Build history of the part. All positions in model axes, mm. A direction names the side the tool comes from. Round coordinates to 2 decimals unless told otherwise and drop trailing zeros. Order: outer loops, then holes, each group sorted by start corner. A loop starts at its lowest first (then second) coordinate and runs counter-clockwise, first axis right, second up. Notation, with made-up numbers: (55.25, 58.5) -> (62.25, 58.5) arc R27 ccw to (62.25, 86.5) -> close; hole circle Ø2 at (63.25, 68). An arc over 180 degrees is marked (long way). Write item = value, one per line.
from build123d import *

# Parameters (mm, degrees)
F1_DEPTH  = 125
F2_R      = 26.25
F3_DEPTH  = 25
F4_W      = 97.6103432477
F4_H      = 17.1008444879
F5_DEPTH  = 22.5
F7_DEPTH  = 223
F9_DEPTH  = 25
F10_R     = 5
F12_DEPTH = 25


with BuildPart() as f1:
    # F0 (on Right) → F1 (new body, symmetric)
    with BuildSketch(Plane.YZ):
        with BuildLine():
            Line((150.9032388148, 0), (0, 0))
            Line((0, 0), (0, -3.0000018725))
            Line((0, -3.0000018725), (150.9032388148, -3.0000018725))
            ThreePointArc((150.9032388148, -3.0000018725), (177.0839005299, 9.9108717028), (182.778792891, 38.541028973))
            Line((182.778792891, 38.541028973), (157.1357605543, 134.2421285136))
            ThreePointArc((157.1357605543, 134.2421285136), (145.53968371, 148.6905408156), (127.0530008041, 149.9022220292))
            Line((127.0530008041, 149.9022220292), (-35.6771693401, 90.6732838797))
            ThreePointArc((-35.6771693401, 90.6732838797), (-44.8528287691, 91.0739018222), (-51.0577201094, 97.8453524901))
            Line((-51.0577201094, 97.8453524901), (-52.767820826, 102.543815594))
            Line((-52.767820826, 102.543815594), (-55.586900448, 101.5177545236))
            Line((-55.586900448, 101.5177545236), (-53.8767997313, 96.8192914196))
            ThreePointArc((-53.8767997313, 96.8192914196), (-46.1206843457, 88.354976764), (-34.6511082697, 87.8542042577))
            Line((-34.6511082697, 87.8542042577), (128.0790618745, 147.0831424073))
            ThreePointArc((128.0790618745, 147.0831424073), (144.1544370057, 146.0295066551), (154.2379812668, 133.4656708936))
            Line((154.2379812668, 133.4656708936), (179.8810136034, 37.7645713531))
            ThreePointArc((179.8810136034, 37.7645713531), (174.7038390235, 11.7371571297), (150.9032388148, 0))
        make_face()
    extrude(amount=F1_DEPTH, both=True)

    # F2 (on face) → F3 (cut)
    with BuildSketch(Plane(origin=(0, 180.1701926471, 48.2764576199), x_dir=(-1, 0, 0), z_dir=(0, 0.9659258263, 0.2588190451))):
        with Locations((0, 35)):
            Circle(F2_R)
    extrude(amount=-F3_DEPTH, mode=Mode.SUBTRACT)

    # F4 (on face) → F5 (cut, symmetric)
    with BuildSketch(Plane(origin=(0, -33.3152677142, 91.5329457678), x_dir=(1, 0, 0), z_dir=(0, -0.3420201433, 0.9396926208))):
        with Locations((93.8051716238, -11.063905455)):
            Rectangle(F4_W, F4_H)
        with Locations((-93.8051716238, -11.063905455)):
            Rectangle(F4_W, F4_H)
    extrude(amount=F5_DEPTH, both=True, mode=Mode.SUBTRACT)

    # F6 (on face) → F7 (cut)
    with BuildSketch(Plane(origin=(0, -33.3152677142, 91.5329457678), x_dir=(1, 0, 0), z_dir=(0, -0.3420201433, 0.9396926208))):
        with BuildLine():
            Line((-124.9454884285, 11.1526290369), (-110, 170.6603467676))
            Line((-110, 170.6603467676), (-107.1620267497, 200.9489946296))
            Line((-107.1620267497, 200.9489946296), (-152.5835648179, 200.9489946296))
            Line((-152.5835648179, 200.9489946296), (-152.5835648179, -22.4528324986))
            Line((-152.5835648179, -22.4528324986), (-112.5, -22.4528324986))
            Line((-112.5, -22.4528324986), (-112.5, -2.5134832111))
            ThreePointArc((-112.5, -2.5134832111), (-121.74192629, 1.5700568176), (-124.9454884285, 11.1526290369))
        make_face()
        with BuildLine():
            Line((112.5, -2.5134832111), (112.5, -22.4528324986))
            Line((112.5, -22.4528324986), (152.5835648179, -22.4528324986))
            Line((152.5835648179, -22.4528324986), (152.5835648179, 200.9489946296))
            Line((152.5835648179, 200.9489946296), (107.1620267497, 200.9489946296))
            Line((107.1620267497, 200.9489946296), (110, 170.6603467676))
            Line((110, 170.6603467676), (124.9454884285, 11.1526290369))
            ThreePointArc((124.9454884285, 11.1526290369), (121.74192629, 1.5700568176), (112.5, -2.5134832111))
        make_face()
    extrude(amount=-F7_DEPTH, mode=Mode.SUBTRACT)

    # F8 (on face) → F9 (cut)
    with BuildSketch(Plane(origin=(0, 0, -3.0000018725), x_dir=(1, 0, 0), z_dir=(0, 0, -1))):
        with BuildLine():
            ThreePointArc((-124.7078686175, -15), (-120.3144703352, -4.3933982822), (-109.7078686175, 0))
            Line((-109.7078686175, 0), (-109.7078686175, 1.8405353206))
            Line((-109.7078686175, 1.8405353206), (-139.135748148, 2.5484173093))
            Line((-139.135748148, 2.5484173093), (-139.135748148, -15))
            Line((-139.135748148, -15), (-124.7078686175, -15))
        make_face()
        with BuildLine():
            Line((109.7078686175, 1.8405353206), (109.7078686175, 0))
            ThreePointArc((109.7078686175, 0), (120.3144703352, -4.3933982822), (124.7078686175, -15))
            Line((124.7078686175, -15), (139.135748148, -15))
            Line((139.135748148, -15), (139.135748148, 2.5484173093))
            Line((139.135748148, 2.5484173093), (109.7078686175, 1.8405353206))
        make_face()
    extrude(amount=-F9_DEPTH, mode=Mode.SUBTRACT)

    # F10
    f10_edges = [f1.edges().sort_by_distance(p)[0] for p in [
        (-45, -35.164139, 89.263744),
        (45, -35.164139, 89.263744),
        (45, -54.177361, 102.030785),
        (-45, -54.177361, 102.030785),
    ]]
    fillet(f10_edges, radius=F10_R)

    # F11 (on face) → F12 (cut)
    with BuildSketch(Plane(origin=(0, -33.3152677142, 91.5329457678), x_dir=(1, 0, 0), z_dir=(0, -0.3420201433, 0.9396926208))):
        with BuildLine():
            ThreePointArc((-9.5571116428, 97.9430625287), (-8.0445828135, 89.0599084724), (0, 85))
            ThreePointArc((0, 85), (8.0445828135, 89.0599084724), (9.5571116428, 97.9430625287))
            add(Edge.make_bspline(
                [(0.2464486877, 118.196647138), (1.8167264508, 108.9800336214), (7.4531598076, 104.7753001668), (9.5571116428, 97.9430625287)],
                knots=[1.4245432684, 1.4245432684, 1.4245432684, 1.4245432684, 24.0384457394, 24.0384457394, 24.0384457394, 24.0384457394], degree=3))
            ThreePointArc((0.2464486877, 118.196647138), (0, 118.4046585168), (-0.2464486877, 118.196647138))
            add(Edge.make_bspline(
                [(-0.2464486877, 118.196647138), (-1.8167264508, 108.9800336214), (-7.4531598076, 104.7753001668), (-9.5571116428, 97.9430625287)],
                knots=[1.4245432684, 1.4245432684, 1.4245432684, 1.4245432684, 24.0384457394, 24.0384457394, 24.0384457394, 24.0384457394], degree=3))
        make_face()
    extrude(amount=-F12_DEPTH, mode=Mode.SUBTRACT)


solid = f1.part
Q1. Cut at A-A, the plane y = 32.5. List the corners of the cut face in (x, z).
Check values:
outline = (-123.23, -3) -> (123.23, -3) -> (123.13, 0) -> (-123.13, 0) -> close; (-119.53, 112.3) -> (119.53, 112.3) -> (119.43, 115.49) -> (-119.43, 115.49) -> close
Q2. Which spindle directions (+Z, -Z, +X, -X, +Y, -Y) get a long thin tool onto all of the face, cutting with end or side? Do faces 1 (the face through (-120.43, 4.51, -1.52)), 2 (the face through (1.578, 174.936, 12.044)), 3 (the face through (1.75, 45.575, 117.054)). Say none if no direction does.
Check values:
face_1 = -Z, -X, -Y
face_2 = +X, -X, -Y
face_3 = +X, -X
Q3. Cut at B-B, the plane x = 23. List the corners of the cut face in (y, z), and give its area (3 significant figures).
Check values:
outline = (-55.59, 101.52) -> (-53.88, 96.82) arc R15 ccw to (-34.65, 87.85) -> (128.08, 147.08) arc R20 cw to (154.24, 133.47) -> (164.94, 93.53) -> (167.84, 94.3) -> (157.14, 134.24) arc R23 ccw to (127.05, 149.9) -> (-35.68, 90.67) arc R12 cw to (-51.06, 97.85) -> (-52.77, 102.54) -> close; (0, -3) -> (150.9, -3) arc R33 ccw to (182.78, 38.54) -> (174.39, 69.86) -> (171.49, 69.09) -> (179.88, 37.76) arc R30 cw to (150.9, 0) -> (0, 0) -> close
area = 1,550 mm²
Q4. Cut at C-C, the plane x = -58. List the corners of the cut face in (y, z), and give its area (3 significant figures).
Check values:
outline = (-35.68, 90.67) -> (-34.65, 87.85) -> (128.08, 147.08) arc R20 cw to (154.24, 133.47) -> (179.88, 37.76) arc R30 cw to (150.9, 0) -> (0, 0) -> (0, -3) -> (150.9, -3) arc R33 ccw to (182.78, 38.54) -> (157.14, 134.24) arc R23 ccw to (127.05, 149.9) -> close
area = 1,550 mm²
Q5. Mould opens along Y. For faces 4 (the face through (120.2, 4.28, -1.52)), 5 (the face through (-45, -47, 92)), 6 (the face through (25.668, 167.288, 96.355)), 7 (the face through (1.54, 143.948, 146.135)) say: released by +Y, released by -Y, zero draft, split by the parting line, or undercut.
Check values:
face_4 = released by -Y
face_5 = zero draft
face_6 = released by +Y
face_7 = undercut
Q6. Cut at D-D, the plane y = 107. List the corners of the cut face in (x, z).
Check values:
outline = (-116.67, -3) -> (116.67, -3) -> (116.57, 0) -> (-116.57, 0) -> close; (-112.1, 139.41) -> (112.1, 139.41) -> (112, 142.6) -> (-112, 142.6) -> close
Q7. Flat gauge pins, fed straight in: pin 1 (1.5 mm diameter, centred on x = 31, y = -18, fed in from -Z); pin 2 (1.5 mm diameter, centred on x = -1.5, z = -2, fed in from -Y); pin 3 (12 mm diameter, centred on y = -48, z = 90, fed in from +X). Where does each tip first touch, or does it go through?
Check values:
pin_1 = 93.64
pin_2 = 0
pin_3 = 45
Q8. Probe probe 1 along Z at (x, y) = (28, 5); probe 2 along Z at (x, y) = (-33.5, 54); probe 3 along Z at (x, y) = (34.5, -46). List the from-to ranges inside material, lowest first.
Check values:
probe_1 = -3 to 0, 102.29 to 105.48
probe_2 = -3 to 0, 120.12 to 123.31
probe_3 = 88.3 to 91.69
